Verification items for this drawing (mm, ordinates from the low corner). A direction names the side the tool comes from. Round coordinates to 2 decimals unless told otherwise and drop trailing zeros. Order: outer loops, then holes, each group sorted by start corner. A loop starts at its lowest first (then second) coordinate and runs counter-clockwise, first axis right, second up.
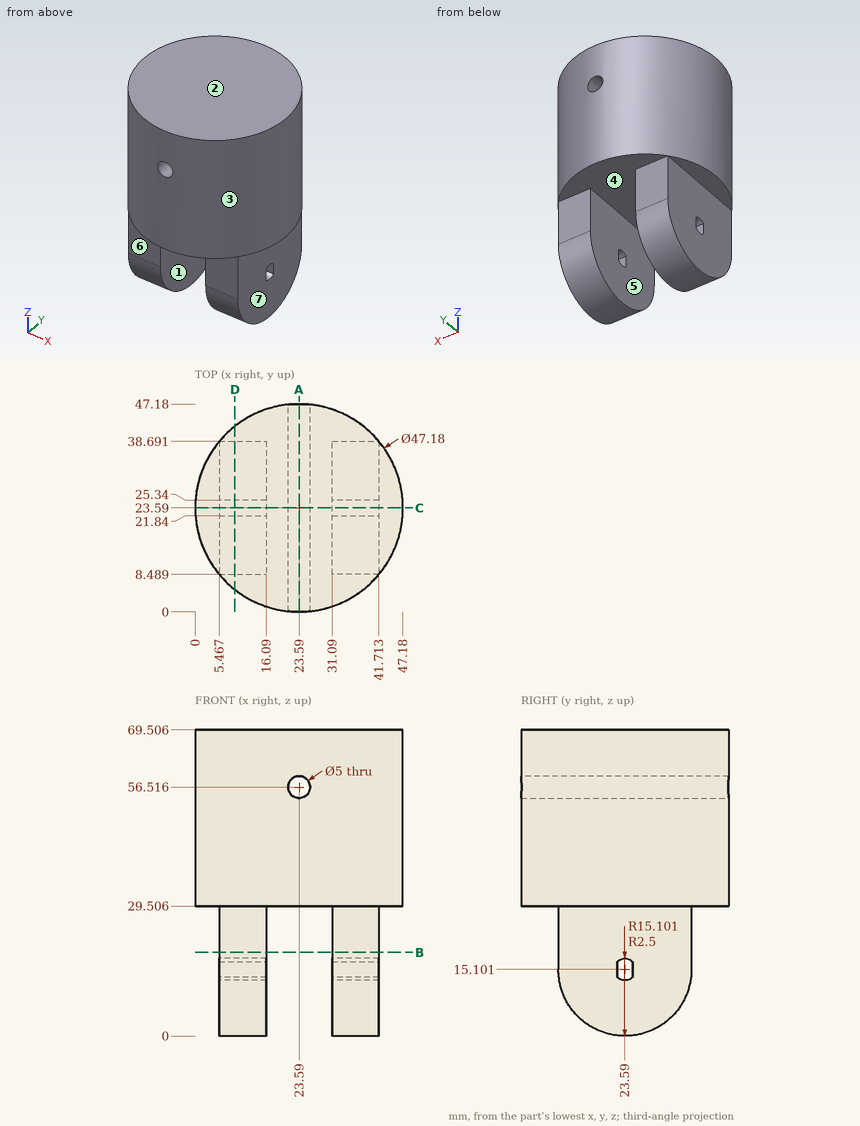
Item 1: Scan lines: line 1 along X through (y, z) = (34, 12.5); line 2 along Z through (x, y) = (21, 15); line 3 along Z through (x, y) = (23, 34). Record each from-to range of solid material in increasing order.
Answer:
line 1: x = 5.47 to 16.09, 31.09 to 41.71
line 2: z = 29.51 to 69.51
line 3: z = 29.51 to 54.09, 58.95 to 69.51
Item 2: Sectioned sample at B-B (z = 19). Record the cut outline in (x, y).
Answer:
outline: (5.47, 8.49) - (16.09, 8.49) - (16.09, 38.69) - (5.47, 38.69) - close; (31.09, 8.49) - (41.71, 8.49) - (41.71, 38.69) - (31.09, 38.69) - close
Item 3: Release check for a two-part mould opening along X. For the marked faces 1, 2, 3 and 4 record: released by +X, released by -X, zero draft, split by the parting line, or undercut.
Answer:
face 1: undercut
face 2: zero draft
face 3: split by the parting line
face 4: undercut
Item 4: Go/stop test with flat-tipped pins: P1, Ø3, axis at y = 12, z = 61, coming from the -X side; P2, Ø3, axis at y = 36, z = 43, coming from the +X side; P3, Ø8.5, axis at x = 9, z = 19.5, coming from the -Y side; P4, Ø12, axis at x = 23, z = 16, coming from the -Y side (1 decimal). Record where each tip stops, or that it passes through.
Answer:
P1: stops at x = 2.27
P2: stops at x = 44.51
P3: stops at y = 8.49
P4: passes through
Item 5: Sectioned sample at C-C (y = 23.59). Record the cut outline in (x, z).
Answer:
outline: (0, 29.51) - (5.47, 29.51) - (5.47, 17.6) - (16.09, 17.6) - (16.09, 29.51) - (31.09, 29.51) - (31.09, 17.6) - (41.71, 17.6) - (41.71, 29.51) - (47.18, 29.51) - (47.18, 69.51) - (0, 69.51) - close; (5.47, 0) - (16.09, 0) - (16.09, 12.6) - (5.47, 12.6) - close; (31.09, 0) - (41.71, 0) - (41.71, 12.6) - (31.09, 12.6) - close; hole circle Ø5 at (23.59, 56.52)
Item 6: Access from +Z, -Z, +X, -X, +Y, -Y to the whole of each face (thin tool, end or side, straight path). Record for the marked faces 5, 6 and 7.
Answer:
face 5: -Z, +Y, -Y
face 6: -Z, +X, -X, -Y
face 7: -Z, +X, +Y, -Y
Item 7: Sectioned sample at A-A (x = 23.59). Record the cut outline in (y, z).
Answer:
outline: (0, 29.51) - (47.18, 29.51) - (47.18, 54.02) - (0, 54.02) - close; (0, 59.02) - (47.18, 59.02) - (47.18, 69.51) - (0, 69.51) - close
Item 8: Sectioned sample at D-D (x = 9). Record the cut outline in (y, z), and give its area (3 significant figures).
Answer:
outline: (5.05, 29.51) - (8.49, 29.51) - (8.49, 15.1) arc R15.1 ccw to (38.69, 15.1) - (38.69, 29.51) - (42.13, 29.51) - (42.13, 69.51) - (5.05, 69.51) - close; hole (21.84, 13.32) arc R2.5 ccw to (25.34, 13.32) - (25.34, 16.89) arc R2.5 ccw to (21.84, 16.89) - close
area: 2,260 mm2
